Input: part model. Units: mm. Frame: model coordinates. A direction names the side the tool comes from. Round coordinates to 2 decimals unless told otherwise and drop trailing zeros. Order: outer loops, then holes, each group sorted by start corner. A loop starts at its lowest first (then second) coordinate and runs counter-clockwise, first axis right, second up. Notation, with made-up numbers: (-37, 61.5) -> (16, 61.5) arc R26 cw to (16, 92.5) -> close; hole circle Ø7 at (86, -30). An arc over 180 degrees is marked (long way). Answer as CSV lines item,"result". Start each with the question number.
1) Section query A-A, the plane x = 5. Output: boundary loops of the cut face in (y, z) (3 decimals), and give its area (3 significant figures).
2) Mould query, pull axis X, two halves, no side actions, for faces 4 (the face through (3.43, -4.74, 42.38)), 5 (the face through (27.861, -2.301, 27.045)), 6 (the face through (36, -5, 38)), 7 (the face through (0, -5, 38)). Classes: +X half, -X half, draft (parallel to the pull), parting line (faces both ways), or undercut.
3) First-contact query: P1, Ø1, axis at x = 7.5, y = -5, coming from the +Z side; P2, Ø0.9, axis at x = 6.5, y = -4.5, coming from the -Z side (3 decimals); P3, Ø1.5, axis at x = 13, y = -4.5, coming from the +Z side. Flat tips, straight axial feed; report the tip coordinate or a pass-through.
4) Section query B-B, the plane y = -4.75. Output: boundary loops of the cut face in (x, z) (1 decimal).
5) Line query: L1, parallel to Z at x = 5, y = -4.5 (3 decimals); L2, parallel to X at y = -5.15, z = 42.25; L3, parallel to Y at x = 9.5, z = 30.75. Output: solid intervals per line, ascending.
6) Access query for faces 1 (the face through (6, -5, 29.975)), 2 (the face through (5.71, -2.3, 30.26)), 3 (the face through (6, -5, 45.975)). Directions: +Z, -Z, +X, -X, +Y, -Y. A direction counts if a zero-diameter tool reaches every point of the face in a straight line with its end or side. Return the directions, or none.
```python
from build123d import *

# Parameters (mm, degrees)
DODANIE_WYCI_GNI_CIE3_DEPTH                      = 4
POG_BIENIE_STO_KOWE_POD_M3_RUB_Z_BEM_D           = 3.4
POG_BIENIE_STO_KOWE_POD_M3_RUB_Z_BEM_DEPTH       = 8
POG_BIENIE_STO_KOWE_POD_M3_RUB_Z_BEM_CSINK_D     = 6.3
POG_BIENIE_STO_KOWE_POD_M3_RUB_Z_BEM_CSINK_ANGLE = 90
POG_BIENIE_STO_KOWE_POD_M3_RUB_Z_BEM_TIP         = 1.021463052
ZAOKR_GLENIE2_R                                  = 4
ZAOKR_GLENIE3_R                                  = 20
ZAOKR_GLENIE4_R                                  = 5
ZAOKR_GLENIE5_R                                  = 1


with BuildPart() as part:
    # Szkic21 → Dodanie-wyci_gni_cie3 (new body)
    with BuildSketch(Plane.XZ.offset(6)):
        Polygon((0, 29.975009918), (10, 29.975009918), (22, 26.759619609), (36, 26.759619609), (36, 49.190400227), (22, 49.190400227), (10, 45.975009918), (0, 45.975009918), align=None)
    extrude(amount=-DODANIE_WYCI_GNI_CIE3_DEPTH)

    # Pog_bienie sto_kowe pod M3 _rub_ z _bem
    with Locations(Plane(origin=(0, -2, 0), x_dir=(1, 0, 0), z_dir=(0, 1, 0))):
        with Locations((5, -41.725009918), (5, -34.225009918)):
            CounterSinkHole(POG_BIENIE_STO_KOWE_POD_M3_RUB_Z_BEM_D / 2, POG_BIENIE_STO_KOWE_POD_M3_RUB_Z_BEM_CSINK_D / 2, depth=POG_BIENIE_STO_KOWE_POD_M3_RUB_Z_BEM_DEPTH, counter_sink_angle=POG_BIENIE_STO_KOWE_POD_M3_RUB_Z_BEM_CSINK_ANGLE)
            with Locations((0, 0, -(POG_BIENIE_STO_KOWE_POD_M3_RUB_Z_BEM_DEPTH + POG_BIENIE_STO_KOWE_POD_M3_RUB_Z_BEM_TIP / 2))):  # 118° drill point
                Cone(0, POG_BIENIE_STO_KOWE_POD_M3_RUB_Z_BEM_D / 2, POG_BIENIE_STO_KOWE_POD_M3_RUB_Z_BEM_TIP, mode=Mode.SUBTRACT)

    # Zaokr_glenie2
    zaokr_glenie2_edges = [part.edges().sort_by_distance(p)[0] for p in [
        (0, -4, 29.975009918),
        (0, -4, 45.975009918),
    ]]
    fillet(zaokr_glenie2_edges, radius=ZAOKR_GLENIE2_R)

    # Zaokr_glenie3
    zaokr_glenie3_edges = [part.edges().sort_by_distance(p)[0] for p in [
        (22, -4, 26.759619609),
        (10, -4, 29.975009918),
        (10, -4, 45.975009918),
        (22, -4, 49.190400227),
    ]]
    fillet(zaokr_glenie3_edges, radius=ZAOKR_GLENIE3_R)

    # Zaokr_glenie4
    zaokr_glenie4_edges = [part.edges().sort_by_distance(p)[0] for p in [
        (36, -4, 26.759619609),
        (36, -4, 49.190400227),
    ]]
    fillet(zaokr_glenie4_edges, radius=ZAOKR_GLENIE4_R)

    # Zaokr_glenie5
    zaokr_glenie5_edges = [part.edges().sort_by_distance(p)[0] for p in [
        (5.683475024, -2, 45.975009918),
        (0, -2, 37.975009918),
        (5.683475024, -2, 29.975009918),
        (1.171572875, -2, 31.146582793),
        (1.171572875, -2, 44.803437043),
        (27.816524976, -2, 49.190400227),
        (16, -2, 47.582705073),
        (27.816524976, -2, 26.759619609),
        (16, -2, 28.367314764),
        (22.022526107, -2, 26.930722382),
        (22.022526107, -2, 49.019297455),
        (9.977473893, -2, 46.146112691),
        (9.977473893, -2, 29.803907146),
        (36, -2, 37.975009918),
        (34.535533906, -2, 28.224085703),
        (34.535533906, -2, 47.725934133),
    ]]
    fillet(zaokr_glenie5_edges, radius=ZAOKR_GLENIE5_R)


solid = part.part
```
Findings:
1,outline,"(-6, 29.975) -> (-3, 29.975) arc R1 ccw to (-2, 30.975) -> (-2, 31.075) -> (-3.45, 32.525) -> (-6, 32.525) -> close; (-6, 35.925) -> (-3.45, 35.925) -> (-2, 37.375) -> (-2, 38.575) -> (-3.45, 40.025) -> (-6, 40.025) -> close; (-6, 43.425) -> (-3.45, 43.425) -> (-2, 44.875) -> (-2, 44.975) arc R1 ccw to (-3, 45.975) -> (-6, 45.975) -> close"
1,area,"32.2 mm^2"
2,face 4,"undercut"
2,face 5,"draft"
2,face 6,"+X half"
2,face 7,"-X half"
3,P1,"stops at z = 45.99"
3,P2,"stops at z = 29.975"
3,P3,"stops at z = 46.98"
4,outline,"(0, 34) arc R4 ccw to (4, 30) -> (7.4, 30) arc R20 cw to (12.5, 29.3) -> (19.5, 27.4) arc R20 ccw to (24.6, 26.8) -> (31, 26.8) arc R5 ccw to (36, 31.8) -> (36, 44.2) arc R5 ccw to (31, 49.2) -> (24.6, 49.2) arc R20 ccw to (19.5, 48.5) -> (12.5, 46.7) arc R20 cw to (7.4, 46) -> (4, 46) arc R4 ccw to (0, 42) -> close; hole circle Ø3.4 at (5, 34.2); hole circle Ø3.4 at (5, 41.7)"
5,L1,"z = 29.975 to 32.525, 35.925 to 40.025, 43.425 to 45.975"
5,L2,"x = 0.01 to 3.38, 6.62 to 36"
5,L3,"y = -6 to -2.01"
6,face 1,"-Z, -X, +Y, -Y"
6,face 2,"-Z, -X, +Y"
6,face 3,"+Z, -X, +Y, -Y"
